Source: CAD feature listing. Evaluate the final solid. Frame: model axes, mm. Face numbers are marked on the shaded views. Round coordinates to 2 decimals unless told otherwise and drop trailing zeros. Loops run counter-clockwise (first coordinate to the right, second up) from the corner with the lowest first, then second, coordinate; pieces in that order, holes last. Notation, with made-up numbers: (-16, 65.25) -> (19, 65.25) arc R15 cw to (19, 94.25) -> close; hole circle Ø5 at (37.25, 13). An arc over 180 degrees is marked (long way). Put each result on its own line as item: value. Start each with the question number.
1. Cut plane C-C (x = -1.25). Return the cut outline in (y, z), then the cut area to 3 significant figures.
2. Material intervals for L1, parallel to Z at x = 0, y = -1.35; L2, parallel to X at y = -2.8, z = -0.5; L3, parallel to Z at x = -1.25, y = -1.4, sorted ascending.
3. Draft query along Z for the marked faces 1, 2 and 3. Return one class per face: pulls with the +Z half, pulls with the -Z half, needs draft (parallel to the pull), parting line crosses it, or undercut.
4. Cut plane D-D (z = -1.25). Return the cut outline in (x, y), then the cut area to 3 significant figures.
5. Cut plane A-A (y = -0.4). Return the cut outline in (x, z), then the cut area to 3 significant figures.
6. Cut plane B-B (z = 1). Return the cut outline in (x, y).
7. Contact query for a flat-ended pin moving along its axis: pin 1 (1 mm diameter, centred on x = -1.5, y = -0.5, fed in from +Z). Output: stop coordinate, or through.
```python
from build123d import *

# Parameters (mm, degrees)
F0_R     = 1.5
F1_DEPTH = 3


with BuildPart() as f1:
    # F0 (on Front) → F1 (new body)
    with BuildSketch(Plane.XZ):
        Circle(F0_R)
        with BuildLine():
            ThreePointArc((0, -4), (2.828427, -2.828427), (4, 0))
            ThreePointArc((4, 0), (2.828427, 2.828427), (0, 4))
            ThreePointArc((0, 4), (-4, 0), (0, -4))
        make_face()
        Circle(F0_R, mode=Mode.SUBTRACT)
        with BuildLine():
            ThreePointArc((0, 4), (2.828427, 2.828427), (4, 0))
            ThreePointArc((4, 0), (5.171573, 2.828427), (8, 4))
            Line((8, 4), (0, 4))
        make_face()
        with BuildLine():
            ThreePointArc((9.5, 0), (8, 1.5), (6.5, 0))
            ThreePointArc((6.5, 0), (8, -1.5), (9.5, 0))
        make_face()
        with BuildLine():
            ThreePointArc((8, 4), (5.171573, 2.828427), (4, 0))
            ThreePointArc((4, 0), (5.171573, -2.828427), (8, -4))
            ThreePointArc((8, -4), (10.828427, -2.828427), (12, 0))
            ThreePointArc((12, 0), (10.828427, 2.828427), (8, 4))
        make_face()
        with BuildLine():
            ThreePointArc((9.5, 0), (8, -1.5), (6.5, 0))
            ThreePointArc((6.5, 0), (8, 1.5), (9.5, 0))
        make_face(mode=Mode.SUBTRACT)
        with BuildLine():
            ThreePointArc((8, -4), (5.171573, -2.828427), (4, 0))
            ThreePointArc((4, 0), (2.828427, -2.828427), (0, -4))
            Line((0, -4), (8, -4))
        make_face()
    extrude(amount=F1_DEPTH)


solid = f1.part
```
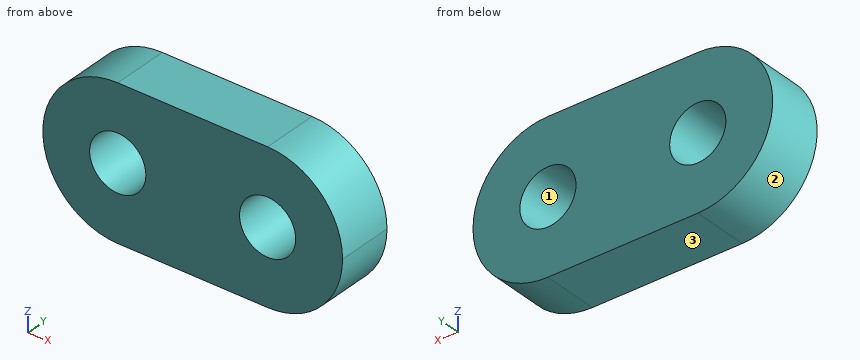
Solution:
1. outline: (-3, -3.8) -> (0, -3.8) -> (0, -0.83) -> (-3, -0.83) -> close; (-3, 0.83) -> (0, 0.83) -> (0, 3.8) -> (-3, 3.8) -> close
1. area: 17.8 mm^2
2. L1: z = -4 to -1.5, 1.5 to 4
2. L2: x = -3.97 to -1.41, 1.41 to 6.59, 9.41 to 11.97
2. L3: z = -3.8 to -0.83, 0.83 to 3.8
3. face 1: undercut
3. face 2: parting line crosses it
3. face 3: pulls with the -Z half
4. outline: (-3.8, -3) -> (-0.83, -3) -> (-0.83, 0) -> (-3.8, 0) -> close; (0.83, -3) -> (7.17, -3) -> (7.17, 0) -> (0.83, 0) -> close; (8.83, -3) -> (11.8, -3) -> (11.8, 0) -> (8.83, 0) -> close
4. area: 36.8 mm^2
5. outline: (0, -4) -> (8, -4) arc R4 ccw to (8, 4) -> (0, 4) arc R4 ccw to start; hole circle Ø3 at (0, 0); hole circle Ø3 at (8, 0)
5. area: 100 mm^2
6. outline: (-3.87, -3) -> (-1.12, -3) -> (-1.12, 0) -> (-3.87, 0) -> close; (1.12, -3) -> (6.88, -3) -> (6.88, 0) -> (1.12, 0) -> close; (9.12, -3) -> (11.87, -3) -> (11.87, 0) -> (9.12, 0) -> close
7. pin 1: stops at z = 3.87
